Design review of the part built by this model. Coordinates are the model's own, in mm. A direction names the side the tool comes from. Give positions to 0.01 mm unless a question says otherwise; leave off trailing zeros. Write each loop counter-clockwise with the first axis right and the second up, starting at its lowest first coordinate (ties: lowest second). Pieces come first, ordered by that corner, then holes. Notation, with made-up numbers: (-14.75, -5.5) -> (28.25, -5.5) arc R10 cw to (28.25, 6.5) -> close; hole circle Ø6 at (11.5, -16.5). An arc over 180 degrees is marked (long way). Put each result on its own line as item: value. Start each with the question number.
from build123d import *

# Parameters (mm, degrees)
F1_DEPTH  = 8
F2_W      = 49.5291427062
F2_H      = 45.9777747887
F3_DEPTH  = 5
F5_DEPTH  = 12
F6_W      = 2.5
F6_H      = 5
F7_DEPTH  = 29.7655713531
F9_DEPTH  = 12
F10_W     = 2.5
F10_H     = 5
F11_DEPTH = 29.7655713531


with BuildPart() as f1:
    # F0 (on Front) → F1 (new body)
    with BuildSketch(Plane.XZ):
        with BuildLine():
            ThreePointArc((15, 0), (0, -15), (-15, 0))
            Line((-15, 0), (-22.7645713531, 28.9777747887))
            Line((-22.7645713531, 28.9777747887), (-24.7645713531, 28.9777747887))
            Line((-24.7645713531, 28.9777747887), (-17, 0))
            ThreePointArc((-17, 0), (0, -17), (17, 0))
            Line((17, 0), (24.7645713531, 28.9777747887))
            Line((24.7645713531, 28.9777747887), (22.7645713531, 28.9777747887))
            Line((22.7645713531, 28.9777747887), (15, 0))
        make_face()
    extrude(amount=F1_DEPTH)

    # F2 (on Front) → F3 (join)
    with BuildSketch(Plane.XZ):
        with Locations((0, 5.9888873943)):
            Rectangle(F2_W, F2_H)
    extrude(amount=-F3_DEPTH)

    # F4 (on face) → F5 (join)
    with BuildSketch(Plane(origin=(0, 0, -17), x_dir=(1, 0, 0), z_dir=(0, 0, -1))):
        Polygon((5, 0), (-5, 0), (-5, -3.6), (-24.7645713531, -3.6), (-24.7645713531, -5), (24.7645713531, -5), (24.7645713531, -3.6), (5, -3.6), align=None)
    extrude(amount=F5_DEPTH)

    # F6 (on face) → F7 (cut, through all)
    with BuildSketch(Plane.YZ.offset(5)):
        with Locations((2.35, -23)):
            Rectangle(F6_W, F6_H)
    extrude(amount=-F7_DEPTH, mode=Mode.SUBTRACT)

    # F8 (on face) → F9 (join)
    with BuildSketch(Plane.XY.offset(28.9777747887)):
        Polygon((24.7645713531, 5), (-24.7645713531, 5), (-24.7645713531, 3.6), (-5, 3.6), (-5, 0), (5, 0), (5, 3.6), (24.7645713531, 3.6), align=None)
    extrude(amount=F9_DEPTH)

    # F10 (on face) → F11 (cut, through all)
    with BuildSketch(Plane.YZ.offset(5)):
        with Locations((2.35, 34.9777747887)):
            Rectangle(F10_W, F10_H)
    extrude(amount=-F11_DEPTH, mode=Mode.SUBTRACT)


solid = f1.part
Q1. For pin 1 (6 mm diameter, centred on x = 10.5, z = -19, fed in from -Y); pin 2 (1.1 mm diameter, centred on y = 2.5, z = 33.5, fed in from -X) (3 decimals); pin 3 (6 mm diameter, centred on x = -12.5, y = -0.5, fed in from +Z); pin 4 (1.5 mm diameter, centred on x = -0.5, y = -5, fed in from -Z), all flat-tipped, find the tip position at first contact; note any pin that passes through.
Q2. To check wall thickness, follow probe 1 along Y at (x, z) = (3, -22.5); probe 2 along Z at (x, y) = (0, 2.5); probe 3 along Y at (x, z) = (0, 31.5). State the ranges of each line that lie inside material, in increasing order. Write a range as from..to.
Q3. Machinability: for faces 1 (the face through (-18.83, -3.94, 14.29)), 2 (the face through (5, 0.6, 34.9)), 3 (the face through (0, 1.1, 35)), 4 (the face through (-20.937, -3.944, 14.692)), which of the approach directions +Z, -Z, +X, -X, +Y, -Y give a long, thin tool a straight path to every point of the face, cutting with its end or side? Answer none if there is none.
Q4. Take a section at B-B on x = 0. Give the boundary of the cut face in (y, z).
Q5. Take a section at A-A on y = -0.75. Give the boundary of the cut face in (x, z).
Q6. Mouldability with a two-part tool opening along Z and no side actions: class faces 5 (the face through (0, 1.1, -23)), 6 (the face through (-15, 2, -17)), 7 (the face through (-15, -8, -4)) as +Z half, -Z half, draft (parallel to the pull), parting line (faces both ways), or undercut.
Q7. Take a section at D-D on z = 27. Give the boundary of the cut face in (x, y), then the cut area to 3 significant figures.
Q8. Take a section at C-C on x = 13. Give the boundary of the cut face in (y, z), then the cut area to 3 significant figures.
Result:
1. pin 1: stops at y = 0
1. pin 2: passes through
1. pin 3: stops at z = 28.98
1. pin 4: stops at z = -17
2. probe 1: y = 0..1.1, 3.6..5
2. probe 2: z = -29..-25.5, -20.5..32.48, 37.48..40.98
2. probe 3: y = 0..5
3. face 1: +Z, -Y
3. face 2: +Z, +X, -Y
3. face 3: +X, -X
3. face 4: -Z, -X, -Y
4. outline: (-8, -17) -> (0, -17) -> (0, -29) -> (5, -29) -> (5, 40.98) -> (0, 40.98) -> (0, -15) -> (-8, -15) -> close; hole (1.1, -25.5) -> (3.6, -25.5) -> (3.6, -20.5) -> (1.1, -20.5) -> close; hole (1.1, 32.48) -> (3.6, 32.48) -> (3.6, 37.48) -> (1.1, 37.48) -> close
5. outline: (-24.76, 28.98) -> (-17, 0) arc R17 ccw to (17, 0) -> (24.76, 28.98) -> (22.76, 28.98) -> (15, 0) arc R15 cw to (-15, 0) -> (-22.76, 28.98) -> close
6. face 5: undercut
6. face 6: -Z half
6. face 7: draft
7. outline: (-24.76, 0) -> (-24.23, 0) -> (-24.23, -8) -> (-22.23, -8) -> (-22.23, 0) -> (22.23, 0) -> (22.23, -8) -> (24.23, -8) -> (24.23, 0) -> (24.76, 0) -> (24.76, 5) -> (-24.76, 5) -> close
7. area: 280 mm^2
8. outline: (-8, -10.95) -> (0, -10.95) -> (0, -17) -> (3.6, -17) -> (3.6, -29) -> (5, -29) -> (5, 40.98) -> (3.6, 40.98) -> (3.6, 28.98) -> (0, 28.98) -> (0, -7.48) -> (-8, -7.48) -> close
8. area: 291 mm^2
